```python
from build123d import *

# Parameters (mm, degrees)
MODEL_R                         = 2.7
AUFSATZ_LINEAR_AUSTRAGEN1_DEPTH = 3


with BuildPart() as part:
    # Model → Aufsatz-Linear austragen1 (new body)
    with BuildSketch(Plane.XY):
        with BuildLine():
            Line((16, 102.25), (10, 102.25))
            ThreePointArc((10, 102.25), (2.928932188, 99.321067812), (0, 92.25))
            Line((0, 92.25), (0, 4))
            ThreePointArc((0, 4), (1.171572875, 1.171572875), (4, 0))
            Line((4, 0), (56, 0))
            ThreePointArc((56, 0), (58.828427125, 1.171572875), (60, 4))
            Line((60, 4), (60, 115))
            ThreePointArc((60, 115), (57.071067812, 122.071067812), (50, 125))
            Line((50, 125), (30, 125))
            ThreePointArc((30, 125), (22.928932188, 122.071067812), (20, 115))
            Line((20, 115), (20, 106.25))
            ThreePointArc((20, 106.25), (18.828427125, 103.421572875), (16, 102.25))
        make_face()
        with Locations((40, 76)):
            Circle(MODEL_R, mode=Mode.SUBTRACT)
        with Locations((40, 96)):
            Circle(MODEL_R, mode=Mode.SUBTRACT)
        with BuildLine():
            Line((11, 7.3), (9, 7.3))
            ThreePointArc((9, 7.3), (6.3, 10), (9, 12.7))
            Line((9, 12.7), (11, 12.7))
            ThreePointArc((11, 12.7), (13.7, 10), (11, 7.3))
        make_face(mode=Mode.SUBTRACT)
        with BuildLine():
            Line((31, 7.3), (29, 7.3))
            ThreePointArc((29, 7.3), (26.3, 10), (29, 12.7))
            Line((29, 12.7), (31, 12.7))
            ThreePointArc((31, 12.7), (33.7, 10), (31, 7.3))
        make_face(mode=Mode.SUBTRACT)
        with BuildLine():
            Line((51, 7.3), (49, 7.3))
            ThreePointArc((49, 7.3), (46.3, 10), (49, 12.7))
            Line((49, 12.7), (51, 12.7))
            ThreePointArc((51, 12.7), (53.7, 10), (51, 7.3))
        make_face(mode=Mode.SUBTRACT)
        with BuildLine():
            Line((18.1, 83), (8.9, 83))
            ThreePointArc((8.9, 83), (8.617157288, 83.117157288), (8.5, 83.4))
            Line((8.5, 83.4), (8.5, 85.6))
            ThreePointArc((8.5, 85.6), (8.617157288, 85.882842712), (8.9, 86))
            Line((8.9, 86), (18.1, 86))
            ThreePointArc((18.1, 86), (18.382842712, 85.882842712), (18.5, 85.6))
            Line((18.5, 85.6), (18.5, 83.4))
            ThreePointArc((18.5, 83.4), (18.382842712, 83.117157288), (18.1, 83))
        make_face(mode=Mode.SUBTRACT)
        with BuildLine():
            Line((18.1, 68.25), (8.9, 68.25))
            ThreePointArc((8.9, 68.25), (8.617157288, 68.367157288), (8.5, 68.65))
            Line((8.5, 68.65), (8.5, 70.85))
            ThreePointArc((8.5, 70.85), (8.617157288, 71.132842712), (8.9, 71.25))
            Line((8.9, 71.25), (18.1, 71.25))
            ThreePointArc((18.1, 71.25), (18.382842712, 71.132842712), (18.5, 70.85))
            Line((18.5, 70.85), (18.5, 68.65))
            ThreePointArc((18.5, 68.65), (18.382842712, 68.367157288), (18.1, 68.25))
        make_face(mode=Mode.SUBTRACT)
        with BuildLine():
            Line((44.75, 105.75), (35.25, 105.75))
            ThreePointArc((35.25, 105.75), (34.967157288, 105.867157288), (34.85, 106.15))
            Line((34.85, 106.15), (34.85, 108.35))
            ThreePointArc((34.85, 108.35), (34.967157288, 108.632842712), (35.25, 108.75))
            Line((35.25, 108.75), (44.75, 108.75))
            ThreePointArc((44.75, 108.75), (45.032842712, 108.632842712), (45.15, 108.35))
            Line((45.15, 108.35), (45.15, 106.15))
            ThreePointArc((45.15, 106.15), (45.032842712, 105.867157288), (44.75, 105.75))
        make_face(mode=Mode.SUBTRACT)
    extrude(amount=AUFSATZ_LINEAR_AUSTRAGEN1_DEPTH)


solid = part.part
```
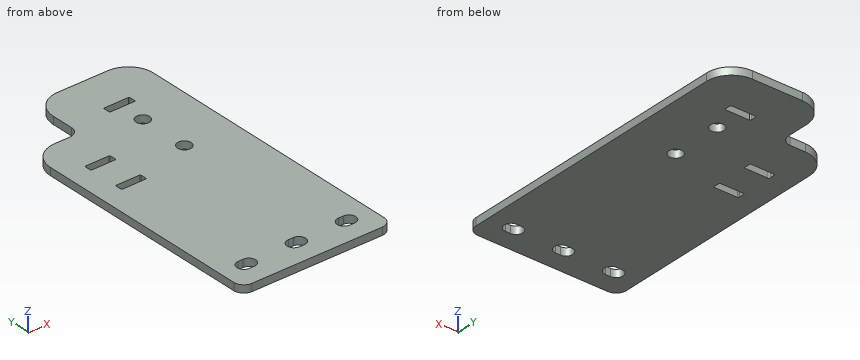
Model file for the job. Use its own axes, mm. Give positions to 0.01 mm unless a question says otherwise; leave off trailing zeros. Order: outer loops, then holes, each group sorted by start corner. A loop starts at its lowest first (then second) coordinate and runs counter-clockwise, first axis right, second up.
1) Wall check: probe 1 along Y at (x, z) = (40, 0.9); probe 2 along Y at (x, z) = (16, 0.9); probe 3 along Y at (x, z) = (50.5, 0.8). Give the ranges that are in metal, low to high.
2) Saw through at D-D, the plane z = 0.65. Count the separate pieces of the cut face and the enclosed holes in it, then the cut area to 3 significant figures.
3) Saw through at B-B, the plane x = 40. Write the cut outline in (y, z), then the cut area to 3 significant figures.
4) Pin check, flat tips, straight feed: pin 1 (1.5 mm diameter, centred on x = 9, z = 1.5, fed in from +Y); pin 2 (5 mm diameter, centred on x = 13.5, y = 103, fed in from +Z). Stop position of each tip, or through.
5) Saw through at C-C, the plane y = 96. Write the cut outline in (x, z).
6) Saw through at A-A, the plane y = 10. Write the cut outline in (x, z).
Computed:
1. probe 1: y = 0 to 73.3, 78.7 to 93.3, 98.7 to 105.75, 108.75 to 125
1. probe 2: y = 0 to 68.25, 71.25 to 83, 86 to 102.25
1. probe 3: y = 0 to 7.3, 12.7 to 124.99
2. separate pieces: 1
2. enclosed holes: 8
2. area: 6,740 mm2
3. outline: (0, 0) - (73.3, 0) - (73.3, 3) - (0, 3) - close; (78.7, 0) - (93.3, 0) - (93.3, 3) - (78.7, 3) - close; (98.7, 0) - (105.75, 0) - (105.75, 3) - (98.7, 3) - close; (108.75, 0) - (125, 0) - (125, 3) - (108.75, 3) - close
3. area: 334 mm2
4. pin 1: stops at y = 102.25
4. pin 2: stops at z = 3
5. outline: (0.73, 0) - (37.3, 0) - (37.3, 3) - (0.73, 3) - close; (42.7, 0) - (60, 0) - (60, 3) - (42.7, 3) - close
6. outline: (0, 0) - (6.3, 0) - (6.3, 3) - (0, 3) - close; (13.7, 0) - (26.3, 0) - (26.3, 3) - (13.7, 3) - close; (33.7, 0) - (46.3, 0) - (46.3, 3) - (33.7, 3) - close; (53.7, 0) - (60, 0) - (60, 3) - (53.7, 3) - close
